Could you check a few things on this model? Use its own coordinates, in mm. Coordinates: 2 decimals unless noted, no trailing zeros. Write each loop counter-clockwise with the first axis right and the second up, starting at its lowest first coordinate (ties: lowest second). Pieces come first, ordered by that corner, then holes. Notation, with made-up numbers: M 65.25,-32 L 119.25,-32 A9 ccw 119.25,-28 Z; hole C -26,89 d9. An arc over 180 degrees is marked long. Write item = value, one per line.
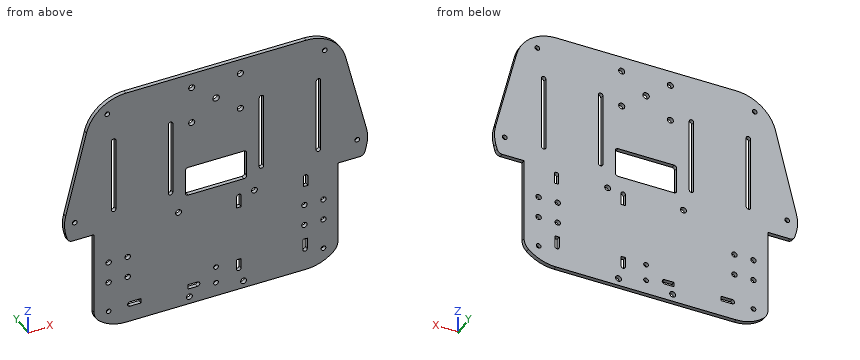
```python
from build123d import *

# Parameters (mm, degrees)
SKETCH_1_R           = 2.414816814
EXTRUDE_1_DEPTH      = 3
SKETCH_2_R           = 1.75
CUT_EXTRUDE_1_DEPTH  = 10
SKETCH_3_R           = 1.75
CUT_EXTRUDE_2_DEPTH  = 10
SKETCH_4_R           = 2
CUT_EXTRUDE_3_DEPTH  = 10
SKETCH_5_R           = 2.187098749
CUT_EXTRUDE_4_DEPTH  = 10
SKETCH_6_R           = 1.75
CUT_EXTRUDE_5_DEPTH  = 10
CUT_EXTRUDE_6_DEPTH  = 10
CUT_EXTRUDE_7_DEPTH  = 10
CUT_EXTRUDE_8_DEPTH  = 10
CUT_EXTRUDE_9_DEPTH  = 10
SKETCH_12_R          = 2.25
CUT_EXTRUDE_10_DEPTH = 10


with BuildPart() as part:
    # 草图1 → 凸台-拉伸1 (new body)
    with BuildSketch(Plane(origin=(0, 0, 0), x_dir=(1, 0, 0), z_dir=(0, 1, 0))):
        with BuildLine():
            Line((90.25, 83.348649636), (90.25, 115.848649636))
            Line((90.25, 115.848649636), (90.25, 131.848649636))
            Line((90.25, 131.848649636), (90.25, 139.378275452))
            ThreePointArc((90.25, 139.378275452), (89.397323186, 143.418879184), (86.984704295, 146.770417094))
            ThreePointArc((86.984704295, 146.770417094), (77.613579276, 152.56980983), (66.78059141, 154.593992167))
            Line((66.78059141, 154.593992167), (-66.78059141, 154.593992167))
            ThreePointArc((-66.78059141, 154.593992167), (-77.613579276, 152.56980983), (-86.984704295, 146.770417094))
            ThreePointArc((-86.984704295, 146.770417094), (-89.397323186, 143.418879184), (-90.25, 139.378275452))
            Line((-90.25, 139.378275452), (-90.25, 131.848649636))
            Line((-90.25, 131.848649636), (-90.25, 83.348649636))
            Line((-90.25, 83.348649636), (-90.25, 76.831438081))
            Line((-90.25, 76.831438081), (-106.330217655, 76.831438081))
            ThreePointArc((-106.330217655, 76.831438081), (-108.765530777, 76.004646236), (-110.194095385, 73.86606308))
            Line((-110.194095385, 73.86606308), (-111.126521712, 70.383853271))
            ThreePointArc((-111.126521712, 70.383853271), (-112.146146857, 62.902573916), (-111.265547961, 55.403659207))
            Line((-111.265547961, 55.403659207), (-95.898700635, -6.566167178))
            ThreePointArc((-95.898700635, -6.566167178), (-85.265515034, -22.974194171), (-66.78059141, -29.345660602))
            Line((-66.78059141, -29.345660602), (66.78059141, -29.345660602))
            ThreePointArc((66.78059141, -29.345660602), (85.265515034, -22.974194171), (95.898700635, -6.566167178))
            Line((95.898700635, -6.566167178), (111.265547961, 55.403659207))
            ThreePointArc((111.265547961, 55.403659207), (112.146146857, 62.902573916), (111.126521712, 70.383853271))
            Line((111.126521712, 70.383853271), (110.194095385, 73.86606308))
            ThreePointArc((110.194095385, 73.86606308), (108.765530777, 76.004646236), (106.330217655, 76.831438081))
            Line((106.330217655, 76.831438081), (90.25, 76.831438081))
            Line((90.25, 76.831438081), (90.25, 83.348649636))
        make_face()
        with Locations(Location((0, -4.151350364, 0), (0, 0, 270))):
            Circle(SKETCH_1_R, mode=Mode.SUBTRACT)
    extrude(amount=EXTRUDE_1_DEPTH)

    # 草图2 → 切除-拉伸1 (cut)
    with BuildSketch(Plane(origin=(0, 3, 0), x_dir=(1, 0, 0), z_dir=(0, 1, 0))):
        with Locations(Location((80.450184708, -16.818951307, 0), (0, 0, 270))):
            Circle(SKETCH_2_R)
        with Locations(Location((104.507530951, 62.624165782, 0), (0, 0, 270))):
            Circle(SKETCH_2_R)
        with Locations(Location((-104.507530951, 62.624165782, 0), (0, 0, 270))):
            Circle(SKETCH_2_R)
        with Locations(Location((-80.450184708, -16.818951307, 0), (0, 0, 270))):
            Circle(SKETCH_2_R)
    extrude(amount=-CUT_EXTRUDE_1_DEPTH, mode=Mode.SUBTRACT)

    # 草图3 → 切除-拉伸2 (cut)
    with BuildSketch(Plane(origin=(0, 3, 0), x_dir=(1, 0, 0), z_dir=(0, 1, 0))):
        with Locations(Location((0, 131.568155221, 0), (0, 0, 270))):
            Circle(SKETCH_3_R)
        with Locations(Location((0, 144.079729864, 0), (0, 0, 270))):
            Circle(SKETCH_3_R)
    extrude(amount=-CUT_EXTRUDE_2_DEPTH, mode=Mode.SUBTRACT)

    # 草图4 → 切除-拉伸3 (cut)
    with BuildSketch(Plane.XZ):
        with Locations(Location((79.5, -102.598649636, 0), (0, 0, 270))):
            Circle(SKETCH_4_R)
        with Locations(Location((65.4, -102.598649636, 0), (0, 0, 270))):
            Circle(SKETCH_4_R)
        with Locations(Location((65.4, -118.598649636, 0), (0, 0, 270))):
            Circle(SKETCH_4_R)
        with Locations(Location((79.5, -118.598649636, 0), (0, 0, 270))):
            Circle(SKETCH_4_R)
        with Locations(Location((-65.4, -102.598649636, 0), (0, 0, 270))):
            Circle(SKETCH_4_R)
        with Locations(Location((-79.5, -102.598649636, 0), (0, 0, 270))):
            Circle(SKETCH_4_R)
        with Locations(Location((-79.5, -118.598649636, 0), (0, 0, 270))):
            Circle(SKETCH_4_R)
        with Locations(Location((-65.4, -118.598649636, 0), (0, 0, 270))):
            Circle(SKETCH_4_R)
    extrude(amount=-CUT_EXTRUDE_3_DEPTH, mode=Mode.SUBTRACT)

    # 草图5 → 切除-拉伸4 (cut)
    with BuildSketch(Plane(origin=(0, 3, 0), x_dir=(1, 0, 0), z_dir=(0, 1, 0))):
        with Locations(Location((28.387774848, 78.93312243, 0), (0, 0, 270))):
            Circle(SKETCH_5_R)
        with Locations(Location((-27.718646552, 78.93312243, 0), (0, 0, 270))):
            Circle(SKETCH_5_R)
        with Locations(Location((20.384564295, 149.11485609, 0), (0, 0, 270))):
            Circle(SKETCH_5_R)
        with Locations(Location((-19.695499635, 149.054892436, 0), (0, 0, 270))):
            Circle(SKETCH_5_R)
    extrude(amount=-CUT_EXTRUDE_4_DEPTH, mode=Mode.SUBTRACT)

    # 草图6 → 切除-拉伸5 (cut)
    with BuildSketch(Plane(origin=(0, 3, 0), x_dir=(1, 0, 0), z_dir=(0, 1, 0))):
        with Locations(Location((79.5, 141.78226533, 0), (0, 0, 270))):
            Circle(SKETCH_6_R)
        with Locations(Location((-79.5, 141.78226533, 0), (0, 0, 270))):
            Circle(SKETCH_6_R)
    extrude(amount=-CUT_EXTRUDE_5_DEPTH, mode=Mode.SUBTRACT)

    # 草图7 → 切除-拉伸6 (cut)
    with BuildSketch(Plane(origin=(0, 3, 0), x_dir=(1, 0, 0), z_dir=(0, 1, 0))):
        with BuildLine():
            Line((67.913857225, 80.150069555), (67.913857225, 87.58815074))
            Line((67.913857225, 87.58815074), (64.613857225, 87.58815074))
            Line((64.613857225, 87.58815074), (64.613857225, 80.150069555))
            ThreePointArc((64.613857225, 80.150069555), (66.263857225, 78.500069555), (67.913857225, 80.150069555))
        make_face()
        with BuildLine():
            Line((18.51822815, 138.15000011), (18.51822815, 130.666323995))
            Line((18.51822815, 130.666323995), (15.21822815, 130.666323995))
            Line((15.21822815, 130.666323995), (15.21822815, 138.15000011))
            ThreePointArc((15.21822815, 138.15000011), (16.86822815, 139.80000011), (18.51822815, 138.15000011))
        make_face()
        with BuildLine():
            Line((18.607981267, 80.150069555), (18.607981267, 88.993926487))
            Line((18.607981267, 88.993926487), (15.307981267, 88.993926487))
            Line((15.307981267, 88.993926487), (15.307981267, 80.150069555))
            ThreePointArc((15.307981267, 80.150069555), (16.957981267, 78.500069555), (18.607981267, 80.150069555))
        make_face()
        with BuildLine():
            Line((64.21822815, 138.15000011), (64.21822815, 129.866807359))
            Line((64.21822815, 129.866807359), (67.51822815, 129.866807359))
            Line((67.51822815, 129.866807359), (67.51822815, 138.15000011))
            ThreePointArc((67.51822815, 138.15000011), (65.86822815, 139.80000011), (64.21822815, 138.15000011))
        make_face()
    extrude(amount=-CUT_EXTRUDE_6_DEPTH, mode=Mode.SUBTRACT)

    # 草图8 → 切除-拉伸7 (cut)
    with BuildSketch(Plane(origin=(0, 3, 0), x_dir=(1, 0, 0), z_dir=(0, 1, 0))):
        with BuildLine():
            Line((-63.718637525, 139.174595172), (-55.596846554, 139.174595172))
            Line((-55.596846554, 139.174595172), (-55.596846554, 142.674595172))
            Line((-55.596846554, 142.674595172), (-63.718637525, 142.674595172))
            ThreePointArc((-63.718637525, 142.674595172), (-65.468637525, 140.924595172), (-63.718637525, 139.174595172))
        make_face()
        with BuildLine():
            Line((-13.718637525, 142.674595172), (-20.649379666, 142.674595172))
            Line((-20.649379666, 142.674595172), (-20.649379666, 139.174595172))
            Line((-20.649379666, 139.174595172), (-13.718637525, 139.174595172))
            ThreePointArc((-13.718637525, 139.174595172), (-11.968637525, 140.924595172), (-13.718637525, 142.674595172))
        make_face()
    extrude(amount=-CUT_EXTRUDE_7_DEPTH, mode=Mode.SUBTRACT)

    # 草图9 → 切除-拉伸8 (cut)
    with BuildSketch(Plane(origin=(0, 3, 0), x_dir=(1, 0, 0), z_dir=(0, 1, 0))):
        with BuildLine():
            Line((-20.688628359, 67.186553007), (20.688628359, 67.186553007))
            ThreePointArc((20.688628359, 67.186553007), (22.102841921, 66.600766569), (22.688628359, 65.186553007))
            Line((22.688628359, 65.186553007), (22.688628359, 46.991155699))
            ThreePointArc((22.688628359, 46.991155699), (22.102841921, 45.576942137), (20.688628359, 44.991155699))
            Line((20.688628359, 44.991155699), (-20.688628359, 44.991155699))
            ThreePointArc((-20.688628359, 44.991155699), (-22.102841921, 45.576942137), (-22.688628359, 46.991155699))
            Line((-22.688628359, 46.991155699), (-22.688628359, 65.186553007))
            ThreePointArc((-22.688628359, 65.186553007), (-22.102841921, 66.600766569), (-20.688628359, 67.186553007))
        make_face()
    extrude(amount=-CUT_EXTRUDE_8_DEPTH, mode=Mode.SUBTRACT)

    # 草图11 → 切除-拉伸9 (cut)
    with BuildSketch(Plane(origin=(0, 3, 0), x_dir=(1, 0, 0), z_dir=(0, 1, 0))):
        with BuildLine():
            Line((-74.128270021, 61.234629534), (-74.128270021, 6.121895865))
            ThreePointArc((-74.128270021, 6.121895865), (-75.778270021, 4.471895865), (-77.428270021, 6.121895865))
            Line((-77.428270021, 6.121895865), (-77.428270021, 61.234629534))
            ThreePointArc((-77.428270021, 61.234629534), (-75.778270021, 62.884629534), (-74.128270021, 61.234629534))
        make_face()
        with BuildLine():
            Line((-31.968935269, 61.234629534), (-31.968935269, 6.121895865))
            ThreePointArc((-31.968935269, 6.121895865), (-33.618935269, 4.471895865), (-35.268935269, 6.121895865))
            Line((-35.268935269, 6.121895865), (-35.268935269, 61.234629534))
            ThreePointArc((-35.268935269, 61.234629534), (-33.618935269, 62.884629534), (-31.968935269, 61.234629534))
        make_face()
        with BuildLine():
            Line((31.968935269, 61.234629534), (31.968935269, 6.121895865))
            ThreePointArc((31.968935269, 6.121895865), (33.618935269, 4.471895865), (35.268935269, 6.121895865))
            Line((35.268935269, 6.121895865), (35.268935269, 61.234629534))
            ThreePointArc((35.268935269, 61.234629534), (33.618935269, 62.884629534), (31.968935269, 61.234629534))
        make_face()
        with BuildLine():
            Line((74.128270021, 61.234629534), (74.128270021, 6.121895865))
            ThreePointArc((74.128270021, 6.121895865), (75.778270021, 4.471895865), (77.428270021, 6.121895865))
            Line((77.428270021, 6.121895865), (77.428270021, 61.234629534))
            ThreePointArc((77.428270021, 61.234629534), (75.778270021, 62.884629534), (74.128270021, 61.234629534))
        make_face()
    extrude(amount=-CUT_EXTRUDE_9_DEPTH, mode=Mode.SUBTRACT)

    # 草图12 → 切除-拉伸10 (cut)
    with BuildSketch(Plane.XZ):
        with Locations(Location((18, 18.151350364, 0), (0, 0, 270))):
            Circle(SKETCH_12_R)
        with Locations(Location((18, -9.848649636, 0), (0, 0, 90))):
            Circle(SKETCH_12_R)
        with Locations(Location((-18, 18.151350364, 0), (0, 0, 90))):
            Circle(SKETCH_12_R)
        with Locations(Location((-18, -9.848649636, 0), (0, 0, 270))):
            Circle(SKETCH_12_R)
    extrude(amount=-CUT_EXTRUDE_10_DEPTH, mode=Mode.SUBTRACT)


solid = part.part
```
Item 1: If I drill on line 1 along X through (y, z) = (1.2, -63); line 2 along X through (y, z) = (0.8, -103); line 3 along X through (y, z) = (0.45, -87), over which ranges is the centre line in solid material (lowest first)?
Numbers:
line_1 = -112.15 to -106.22, -102.8 to -22.69, 22.69 to 102.8, 106.22 to 112.15
line_2 = -90.25 to -81.46, -77.54 to -67.36, -63.44 to 63.44, 67.36 to 77.54, 81.46 to 90.25
line_3 = -90.25 to 15.31, 18.61 to 64.61, 67.91 to 90.25
Item 2: Imagine slicing it at A-A (z = -97). Write out the boundary of the cut face in (x, y), and give its area (4 significant figures).
Numbers:
outline = M -90.25,0 L 90.25,0 L 90.25,3 L -90.25,3 Z
area = 541.5 mm²
Item 3: Imagine slicing it at B-B (y = 0.9). State how many separate pieces and enclosed holes the cut face has, and give its area (3 significant figures).
Numbers:
separate_pieces = 1
enclosed_holes = 36
area = 33,200 mm²
Item 4: I'm going to push flat-ended pins straight in: P1, Ø7, axis at x = 28.39, z = -78.93, coming from the -Y side; P2, Ø3, axis at x = 79.5, z = -141.78, coming from the -Y side; P3, Ø0.9, axis at y = 2, z = -37.5, coming from the -X side. Where does each tip first touch, or does it pass through?
Numbers:
P1 = 0
P2 = through
P3 = -106.94
